Verification items for this drawing (mm, ordinates from the low corner). A direction names the side the tool comes from. Round coordinates to 2 decimals unless told otherwise and drop trailing zeros. Loops run counter-clockwise (first coordinate to the right, second up) from the corner with the lowest first, then second, coordinate; pieces in that order, holes last. Notation, with made-up numbers: (42.25, 19) -> (72.25, 19) arc R12 cw to (72.25, 37) -> close; hole circle Ø8 at (-15, 3). An arc over 180 degrees is marked (long way). One line per item, written item: value. Start each with the question number.
1. Material ranges on L1, parallel to Y at x = 9, z = 32.75; L2, parallel to Z at x = 15, y = 6.5; L3, parallel to X at y = 9.25, z = 11.5, recorded low to high.
2. Release check for a two-part mould opening along X. For the marked faces 3, 4 and 5 record: +X half, -X half, draft (parallel to the pull), parting line (faces both ways), or undercut.
3. Cross-section at C-C on z = 35.5. Record the cut outline in (x, y).
4. Go/stop test with flat-tipped pins: pin 1 (3 mm diameter, centred on x = 9.5, y = 8, fed in from +Z); pin 2 (4 mm diameter, centred on y = 2, z = 13.5, fed in from +X); pin 3 (3 mm diameter, centred on y = 10, z = 32, fed in from +X). Record where each tip stops, or that it passes through.
5. Cross-section at D-D on z = 12. Record the cut outline in (x, y).
6. Set-up check for the marked faces 1 and 2: record each of +Z, -Z, +X, -X, +Y, -Y from which the full face is reachable in a straight line by a thin tool's end or side.
7. Cross-section at A-A on x = 9. Record the cut outline in (y, z).
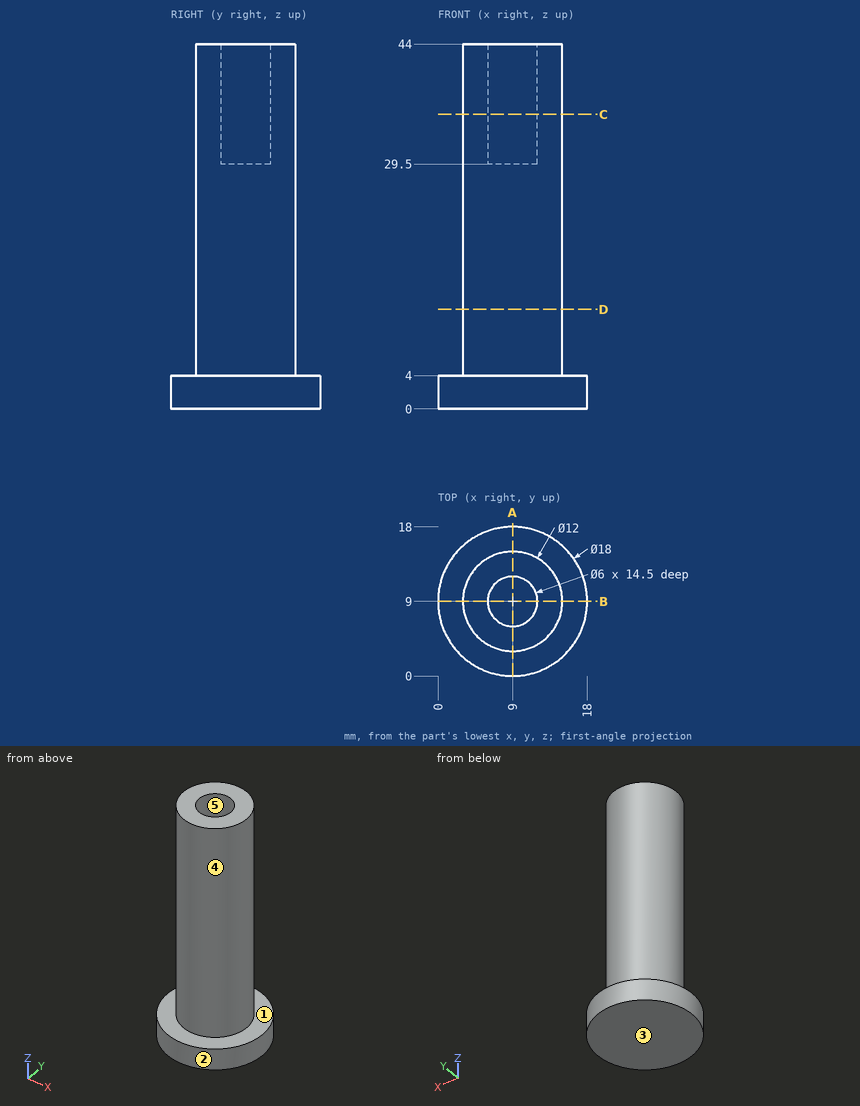
Taken from the geometry:
1. L1: y = 3 to 6, 12 to 15
1. L2: z = 0 to 4
1. L3: x = 3.01 to 14.99
2. face 3: draft
2. face 4: parting line
2. face 5: undercut
3. outline: circle Ø12 at (9, 9); hole circle Ø6 at (9, 9)
4. pin 1: stops at z = 29.5
4. pin 2: stops at x = 12.32
4. pin 3: stops at x = 15
5. outline: circle Ø12 at (9, 9)
6. face 1: +Z
6. face 2: +Z, -Z
7. outline: (0, 0) -> (18, 0) -> (18, 4) -> (15, 4) -> (15, 44) -> (12, 44) -> (12, 29.5) -> (6, 29.5) -> (6, 44) -> (3, 44) -> (3, 4) -> (0, 4) -> close
